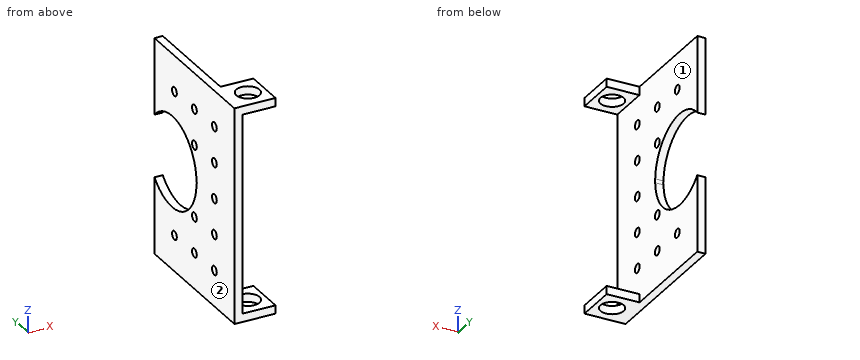
Autodesk Inventor part; units mm, degrees
ref_plane "YZ Plane" through (0, 0, 0) normal (1, 0, 0) x (0, 1, 0)
ref_plane "XZ Plane" through (0, 0, 0) normal (0, 1, 0) x (-1, 0, 0)
ref_plane "XY Plane" through (0, 0, 0) normal (0, 0, 1) x (1, 0, 0)
sketch "Sketch1" plane through (0, 0, 0) normal (1, 0, 0) x (0, 1, 0)
  line L0 (-57.2668, 82.55) -> (-57.2668, -82.55)
  line L1 (-57.2668, -82.55) -> (57.2668, -82.55)
  line L2 (57.2668, -82.55) -> (57.2668, 82.55)
  line L3 (57.2668, 82.55) -> (-57.2668, 82.55)
  line L4 (-57.2668, 82.55) -> (57.2668, -82.55) construction
  line L5 (-57.2668, -82.55) -> (57.2668, 82.55) construction
  line L6 (57.2668, 0) -> (-57.2668, 0) construction
  circle A0 centre (31.8668, 0) radius 34.925
  line L7 (-31.8668, 82.55) -> (-31.8668, -82.55) construction
  point P0 (0, 0)
  point P1 (57.2668, -23.9707)
  point P2 (57.2668, 23.9707)
  dimension "d0" = 165.1
  dimension "d1" = 25.4
  dimension "d2" = 69.85
  dimension "d3" = 63.7337
  dimension "d4" = 25.4
extrude "Extrusion1" add sketch "Sketch1" against normal blind 6.35 contours L3 L2 A0 L1 L0
sketch "Sketch2" plane through (0, 0, 0) normal (1, 0, 0) x (0, 0, -1)
  line L0 (82.55, -57.2668) -> (-82.55, -57.2668)
  line L1 (-82.55, -57.2668) -> (-76.2, -57.2668)
  line L2 (-76.2, -57.2668) -> (-76.2, -25.5168)
  line L3 (-76.2, -25.5168) -> (-82.55, -25.5168)
  line L4 (-82.55, -25.5168) -> (-82.55, -57.2668)
  line L5 (82.55, -57.2668) -> (76.2, -57.2668)
  line L6 (76.2, -57.2668) -> (76.2, -25.5168)
  line L7 (76.2, -25.5168) -> (82.55, -25.5168)
  line L8 (82.55, -25.5168) -> (82.55, -57.2668)
  point P0 (0, 0)
  point P1 (76.2, -57.2668)
  dimension "d7" = 6.35
  dimension "d8" = 6.35
  dimension "d15" = 31.75
extrude "Extrusion2" add sketch "Sketch2" along normal blind 25.2001
sketch "Sketch4" plane through (-6.35, 57.2668, 82.55) normal (0, 0, 1) x (1, 0, 0)
  line L0 (31.5501, -82.7837) -> (31.5501, -114.5337) construction
  line L1 (31.5501, -98.6587) -> (0, -98.6587) construction
  line L2 (0, 0) -> (0, -114.5337) construction
  circle A0 centre (18.8501, -98.6587) radius 8.89
  point P0 (6.35, -57.2668)
  dimension "d11" = 18.8501
  dimension "d12" = 17.78
extrude "Extrusion3" cut sketch "Sketch4" against normal up to surface (6.35 mm away)
sketch "Sketch5" plane through (-6.35, 0, 0) normal (-1, 0, 0) x (0, 0, 1)
  line L0 (-82.55, 57.2668) -> (-82.55, -57.2668)
  line L1 (-82.55, -57.2668) -> (82.55, -57.2668)
  point P0 (0, 0)
  point P1 (-55.0333, -28.6334)
  dimension "d23" = 27.5167
  dimension "d24" = 28.6334
hole "Hole1" at (-6.35, -28.6334, -55.0333) direction (1, 0, 0) diameter 6.7564 end through all
pattern_linear "Rectangular Pattern1" count 3 spacing 28.6334 along (0, 1, 0) count 5 spacing 27.5167 along (0, 0, 1) of "Hole1"
mirror "Mirror2" about plane through (0, 0, 0) normal (0, 0, 1) of "Extrusion3"
equation "\"d0\" = forkWidth"
equation "\"d5\" = wallThickness"
equation "\"d7\" = wallThickness"
equation "\"d8\" = wallThickness"
equation "\"d9\" = centerWormGearAbovePlate + wallThickness"
equation "\"d11\" = centerWormGearAbovePlate"
equation "\"forkWidth\" = 165.1"
equation "\"centerGearToCenterWormGear\" = 73.25868"
equation "\"centerWormGearAbovePlate\" = 18.8501"
equation "\"wallThickness\" = 6.35"
equation "\"widthOfWorm\" = 38.1"
equation "\"holeFor3_8HexShaft\" = 12.7"
properties part number "plateForAzimuthKnobs"
Source: CAD feature listing. Evaluate the final solid. Frame: model axes, mm. Face numbers are marked on the shaded views. Round coordinates to 2 decimals unless told otherwise and drop trailing zeros. Loops run counter-clockwise (first coordinate to the right, second up) from the corner with the lowest first, then second, coordinate; pieces in that order, holes last. Notation, with made-up numbers: M -27.75,12.5 L 20.25,12.5 A35 cw 20.25,48.5 Z; hole C 55.5,34.5 d11. An arc over 180 degrees is marked long. Answer as CSV lines item,"result".
Q1. Contact query for flat-ended pins moving along their axis: pin 1 (7 mm diameter, centred on x = 17.5, z = 79.5, fed in from +Y); pin 2 (9 mm diameter, centred on y = -28.63, z = 55.03, fed in from +X). Output: stop coordinate, or through.
Verdict:
pin 1,"stops at y = -25.52"
pin 2,"stops at x = 0"
Q2. Cut plane B-B (x = 9.5). Return the cut outline in (y, z), plus the area to 3 significant figures.
Verdict:
outline,"M -57.27,-82.55 L -49.76,-82.55 L -49.76,-76.2 L -57.27,-76.2 Z; M -57.27,76.2 L -49.76,76.2 L -49.76,82.55 L -57.27,82.55 Z; M -33.02,-82.55 L -25.52,-82.55 L -25.52,-76.2 L -33.02,-76.2 Z; M -33.02,76.2 L -25.52,76.2 L -25.52,82.55 L -33.02,82.55 Z"
area,"191 mm^2"
Q3. Pull-direction query (Z, two-part tool) for the marked faces 1 and 2; classes: +Z half, -Z half, draft (parallel to the pull), parting line (faces both ways), or undercut.
Verdict:
face 1,"undercut"
face 2,"draft"
Q4. Cut plane D-D (z = -37.5). Return the cut outline in (x, y).
Verdict:
outline,"M -6.35,-57.27 L 0,-57.27 L 0,57.27 L -6.35,57.27 Z"
Q5. Cut plane A-A (y = 0). Count the separate pieces of the cut face and the enclosed holes in it, plus the area to 3 significant figures.
Verdict:
separate pieces,"6"
enclosed holes,"0"
area,"695 mm^2"
Q6. Line query: line 1 along X through (y, z) = (-5, -73.5); line 2 along Z through (x, y) = (-1, 25). Output: solid intervals per line, ascending.
Verdict:
line 1,"x = -6.35 to 0"
line 2,"z = -82.55 to -34.24, 34.24 to 82.55"
Q7. Cut plane C-C (y = 44). Return the cut outline in (x, z).
Verdict:
outline,"M -6.35,-82.55 L 0,-82.55 L 0,-32.75 L -6.35,-32.75 Z; M -6.35,32.75 L 0,32.75 L 0,82.55 L -6.35,82.55 Z"
